from build123d import *

# Parameters (mm, degrees)
F1_DEPTH = 63.5
F2_DEPTH = 25.4
F3_DEPTH = 7.9375


with BuildPart() as f1:
    # F0 (on Front) → F1 (new body, symmetric)
    with BuildSketch(Plane.XZ):
        Polygon((-41.275, -9.525), (41.275, -9.525), (41.275, 9.525), (22.225, 9.525), (-41.275, 9.525), align=None)
    extrude(amount=F1_DEPTH, both=True)

    # F0 (on Front) → F2 (join, symmetric)
    with BuildSketch(Plane.XZ):
        with BuildLine():
            Line((22.225, 9.525), (41.275, 9.525))
            Line((41.275, 9.525), (41.275, 27.0002))
            ThreePointArc((41.275, 27.0002), (45.9246798487, 38.2255201513), (57.15, 42.8752))
            Line((57.15, 42.8752), (60.325, 42.8752))
            Line((60.325, 42.8752), (60.325, 61.9252))
            Line((60.325, 61.9252), (57.15, 61.9252))
            add(Edge.make_bspline(
                [(55.6546739899, 61.8931738647), (56.1494536046, 61.9037814957), (56.6478649939, 61.9144247136), (57.15, 61.9252)],
                knots=[110.1378686708, 110.1378686708, 110.1378686708, 110.1378686708, 111.5045361635, 111.5045361635, 111.5045361635, 111.5045361635], degree=3))
            ThreePointArc((55.6546739899, 61.8931738647), (31.9311589689, 51.1614433879), (22.225, 27.0002))
            Line((22.225, 27.0002), (22.225, 9.525))
        make_face()
    extrude(amount=F2_DEPTH, both=True)

    # F0 (on Front) → F3 (join, symmetric)
    with BuildSketch(Plane.XZ):
        with BuildLine():
            add(Edge.make_bspline(
                [(-41.275, 9.525), (-0.5058915332, 60.4145856104), (15.7810598781, 61.0383193594), (55.6546739899, 61.8931738647)],
                knots=[0, 0, 0, 0, 110.1378686708, 110.1378686708, 110.1378686708, 110.1378686708], degree=3))
            Line((-41.275, 9.525), (22.225, 9.525))
            Line((22.225, 9.525), (22.225, 27.0002))
            ThreePointArc((22.225, 27.0002), (31.9311589689, 51.1614433879), (55.6546739899, 61.8931738647))
        make_face()
    extrude(amount=F3_DEPTH, both=True)


solid = f1.part
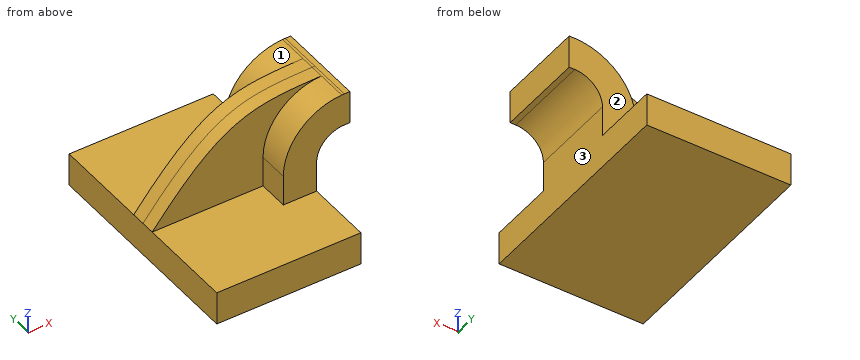
Work out the finished part from the listing and answer in its coordinate system (mm). Face numbers are marked on the shaded views. A direction names the side the tool comes from. Round coordinates to 2 decimals unless told otherwise and drop trailing zeros. Write each loop counter-clockwise with the first axis right and the second up, starting at its lowest first coordinate (ties: lowest second). Pieces come first, ordered by that corner, then holes.
1) A cutting plane is placed at B-B (z = 0.5). Give the vertices of the cut face in (x, y) (3 decimals).
2) A cutting plane is placed at A-A (y = -38). Give the vertices of the cut face in (x, z) (3 decimals), plus the area to 3 significant figures.
3) Given pin 1 Ø5 at (y, z) = (-15, 22.5) entering from -X (3 decimals); pin 2 Ø10 at (y, z) = (-7, 24.5) entering from -X; pin 3 Ø8 at (y, z) = (26.5, 42) entering from -X, each flat-ended and moving along its own axis, determine where each tip first touches the part or whether it passes through.
4) A tool of negligible diameter and unlimited length cuts with its end or side. For the marked faces 1, 2 and 3, from which of +Z, -Z, +X, -X, +Y, -Y can it reach the whole face along a straight path? Write none if from no direction.
5) Straight lines are drawn through the part: line 1 (Z direction, x = 25, y = -58) (3 decimals); line 2 (X direction, y = -23, z = 12) (3 decimals); line 3 (X direction, y = 47, z = 4.5) (3 decimals). For each, find the intervals that lie inside material, in ascending order.
Completed:
1. outline: (-41.275, -63.5) - (41.275, -63.5) - (41.275, 63.5) - (-41.275, 63.5) - close
2. outline: (-41.275, -9.525) - (41.275, -9.525) - (41.275, 9.525) - (-41.275, 9.525) - close
2. area: 1,570 mm2
3. pin 1: stops at x = 22.225
3. pin 2: stops at x = -33.05
3. pin 3: stops at x = 24.05
4. face 1: +Z, -X, +Y
4. face 2: +Z, +X, -X, +Y
4. face 3: -Z, +X, +Y, -Y
5. line 1: z = -9.525 to 9.525
5. line 2: x = 22.225 to 41.275
5. line 3: x = -41.275 to 41.275
